For this review, take the finished solid that the model builds, in its own axes (mm). A direction names the side the tool comes from. Coordinates: 2 decimals unless noted, no trailing zeros. Write each loop counter-clockwise with the first axis right and the second up, starting at its lowest first coordinate (ties: lowest second). Pieces come first, ordered by that corner, then holes. Notation, with made-up numbers: (45.5, 76.5) - (77.5, 76.5) arc R26 cw to (77.5, 105.5) - close; hole circle Ø3 at (-24, 15.25). An arc over 180 degrees is marked (long way). Write each question's results on one line, items separated by ' | '.
from build123d import *

# Parameters (mm, degrees)
SKETCH_1_R          = 4.25
EXTRUDE_1_DEPTH     = 1
SKETCH_2_R          = 7.5
EXTRUDE_2_DEPTH     = 1
SKETCH_3_R          = 1
CUT_EXTRUDE_1_DEPTH = 1
SKETCH_4_R          = 1.5
CUT_EXTRUDE_2_DEPTH = 11.793516572


with BuildPart() as part:
    # 草图1 → 凸台-拉伸1 (new body)
    with BuildSketch(Plane.XY):
        Circle(SKETCH_1_R)
    extrude(amount=EXTRUDE_1_DEPTH)

    # 草图2 → 凸台-拉伸2 (add)
    with BuildSketch(Plane(origin=(0, 0, 0), x_dir=(-1, 0, 0), z_dir=(0, 0, -1))):
        Circle(SKETCH_2_R)
    extrude(amount=EXTRUDE_2_DEPTH)

    # 草图3 → 切除-拉伸1 (cut)
    with BuildSketch(Plane.XY):
        with Locations((6, 0)):
            Circle(SKETCH_3_R)
        with Locations((0, 6)):
            Circle(SKETCH_3_R)
        with Locations((-6, 0)):
            Circle(SKETCH_3_R)
        with Locations((0, -6)):
            Circle(SKETCH_3_R)
    extrude(amount=-CUT_EXTRUDE_1_DEPTH, mode=Mode.SUBTRACT)

    # 草图4 → 切除-拉伸2 (cut, through all)
    with BuildSketch(Plane(origin=(0, 0, -1), x_dir=(-1, 0, 0), z_dir=(0, 0, -1))):
        Circle(SKETCH_4_R)
    extrude(amount=-CUT_EXTRUDE_2_DEPTH, mode=Mode.SUBTRACT)


solid = part.part
Q1. Take a section at B-B on x = 0. State the section outline as (y, z) points.
Results found:
outline: (-7.5, -1) - (-7, -1) - (-7, 0) - (-7.5, 0) - close; (-5, -1) - (-1.5, -1) - (-1.5, 1) - (-4.25, 1) - (-4.25, 0) - (-5, 0) - close; (1.5, -1) - (5, -1) - (5, 0) - (4.25, 0) - (4.25, 1) - (1.5, 1) - close; (7, -1) - (7.5, -1) - (7.5, 0) - (7, 0) - close
Q2. For faces 4 (the face through (-6.8, -0.6, -0.5)), 5 (the face through (-3.2, -3.2, 0)), list the 3-axis set-ups (+Z, -Z, +X, -X, +Y, -Y) from which the entire face can be reached by the end or side of a thin tool; tool diameter is ignored.
Results found:
face 4: +Z, -Z | face 5: +Z
Q3. Mouldability with a two-part tool opening along X and no side actions: class faces 1 (the face through (2.285, 3.584, 0.493)), 2 (the face through (2, 0, 1)), 3 (the face through (1.5, 0.07, -0.01)) as pulls with the +X half, pulls with the -X half, needs draft (parallel to the pull), parting line crosses it, or undercut.
Results found:
face 1: parting line crosses it | face 2: needs draft | face 3: undercut
Q4. Take a section at A-A on y = -6. State the section outline as (x, z) points, plus the area to 3 significant figures.
Results found:
outline: (-4.5, -1) - (-1, -1) - (-1, 0) - (-4.5, 0) - close; (1, -1) - (4.5, -1) - (4.5, 0) - (1, 0) - close | area: 7.00 mm2
Q5. Take a section at C-C on z = -0.3. State the section outline as (x, y) points, plus the area to 3 significant figures.
Results found:
outline: circle Ø15 at (0, 0); hole circle Ø2 at (-6, 0); hole circle Ø3 at (0, 0); hole circle Ø2 at (0, -6); hole circle Ø2 at (0, 6); hole circle Ø2 at (6, 0) | area: 157 mm2
Q6. Wall thickness on line 1 along X through (y, z) = (-6.5, -0.8); line 2 along Y through (x, z) = (6, -0.55); line 3 along Z through (x, y) = (-6.25, -1): over which ranges is each line inside the solid? List them lowest first. Write a range as from..to.
Results found:
line 1: -3.74..-0.87, 0.87..3.74 | line 2: -4.5..-1, 1..4.5 | line 3: -1..0
Q7. For pin 1 (3 mm diameter, centred on x = 0, y = 6, fed in from +Z); pin 2 (3.5 mm diameter, centred on x = 0, y = 0, fed in from -Z), all flat-tipped, find the tip position at first contact; note any pin that passes through.
Results found:
pin 1: z = 0 | pin 2: z = -1
